```python
from build123d import *

# Parameters (mm, degrees)
SKETCH1_R           = 73.66
SKETCH1_R_2         = 6.35
BOSS_EXTRUDE1_DEPTH = 3.175


with BuildPart() as part:
    # Sketch1 → Boss-Extrude1 (new body)
    with BuildSketch(Plane(origin=(0, 0, 0), x_dir=(1, 0, 0), z_dir=(0, 1, 0))):
        with BuildLine():
            Line((12.7, 114.3), (0, 114.3))
            ThreePointArc((0, 114.3), (-69.761055355, 86.634356609), (-101.6, 18.676470588))
            Line((-101.6, 18.676470588), (-101.6, -114.3))
            Line((-101.6, -114.3), (101.6, -114.3))
            Line((101.6, -114.3), (101.6, 25.4))
            ThreePointArc((101.6, 25.4), (75.561792847, 88.261792847), (12.7, 114.3))
        make_face()
        with Locations(Location((0, 6.35, 0), (0, 0, 270))):
            Circle(SKETCH1_R, mode=Mode.SUBTRACT)
        with Locations(Location((-90.060644326, -24.660366712, 0), (0, 0, 270))):
            Circle(SKETCH1_R_2, mode=Mode.SUBTRACT)
        with Locations(Location((-50.8, -101.6, 0), (0, 0, 270))):
            Circle(SKETCH1_R_2, mode=Mode.SUBTRACT)
        with Locations(Location((50.8, -101.6, 0), (0, 0, 90))):
            Circle(SKETCH1_R_2, mode=Mode.SUBTRACT)
        with Locations(Location((18.17455681, 99.849989223, 0), (0, 0, 270))):
            Circle(SKETCH1_R_2, mode=Mode.SUBTRACT)
        with Locations(Location((71.886087516, -56.139622511, 0), (0, 0, 270))):
            Circle(SKETCH1_R_2, mode=Mode.SUBTRACT)
    extrude(amount=BOSS_EXTRUDE1_DEPTH)


solid = part.part
```
Could you check a few things on this model? Use its own coordinates, in mm. Give positions to 0.01 mm unless a question says otherwise; leave off trailing zeros. Write each loop counter-clockwise with the first axis right and the second up, starting at its lowest first coordinate (ties: lowest second). Pieces come first, ordered by that corner, then holes. Notation, with made-up numbers: (-4.75, -4.5) - (33.25, -4.5) arc R18 ccw to (33.25, 19.5) - close; hole circle Ø4 at (46, -25.5). An arc over 180 degrees is marked (long way). One line per item, written item: value. Start each with the question number.
Item 1: If we mould it in two halves opening along X, with no side actions, what happens to faces 1 (the face through (-68.97, 1.57, -87.37)), 2 (the face through (50.521, 1.565, 107.944)), 3 (the face through (76.249, 1.565, -87.567))? For each: +X half, -X half, draft (parallel to the pull), parting line (faces both ways), or undercut.
Item 2: Imagine slicing it at B-B, the plane x = -50.8. List the corners of the cut face in (y, z) for me (3 decimals).
Item 3: I'm going to push a flat-ended pin straight in: pin 1 (16.5 mm diameter, centred on x = 50.8, z = 101.6, fed in from +Y) (3 decimals). Where does the tip first touch, or does it pass through?
Item 4: Imagine slicing it at A-A, the plane z = 101.6. List the corners of the cut face in (x, y) for me (3 decimals).
Item 5: Imagine slicing it at C-C, the plane z = -6.35. List the corners of the cut face in (x, y) for me (3 decimals).
Item 6: Please list where these lines run through material, in increasing order: line 1 (X direction, y = 0.8, z = -6.35); line 2 (X direction, y = 1.5, z = 59.5); line 3 (X direction, y = 0.5, z = 60). Write a range as from..to.
Item 7: Imagine slicing it at D-D, the plane x = 62. List the corners of the cut face in (y, z) for me (3 decimals), and give its area (3 significant figures).
Geometry says:
1. face 1: -X half
1. face 2: undercut
1. face 3: +X half
2. outline: (0, -100.717) - (3.175, -100.717) - (3.175, -59.69) - (0, -59.69) - close; (0, 46.99) - (3.175, 46.99) - (3.175, 95.25) - (0, 95.25) - close; (0, 107.95) - (3.175, 107.95) - (3.175, 114.3) - (0, 114.3) - close
3. pin 1: y = 3.175
4. outline: (-101.6, 0) - (-57.15, 0) - (-57.15, 3.175) - (-101.6, 3.175) - close; (-44.45, 0) - (44.45, 0) - (44.45, 3.175) - (-44.45, 3.175) - close; (57.15, 0) - (101.6, 0) - (101.6, 3.175) - (57.15, 3.175) - close
5. outline: (-101.6, 0) - (-73.66, 0) - (-73.66, 3.175) - (-101.6, 3.175) - close; (73.66, 0) - (101.6, 0) - (101.6, 3.175) - (73.66, 3.175) - close
6. line 1: -101.6..-73.66, 73.66..101.6
6. line 2: -101.6..-33.01, 33.01..66.5, 77.27..101.6
6. line 3: -101.6..-31.99, 31.99..66.84, 76.93..101.6
7. outline: (0, -99.378) - (3.175, -99.378) - (3.175, -46.122) - (0, -46.122) - close; (0, 33.422) - (3.175, 33.422) - (3.175, 114.3) - (0, 114.3) - close
7. area: 426 mm^2
